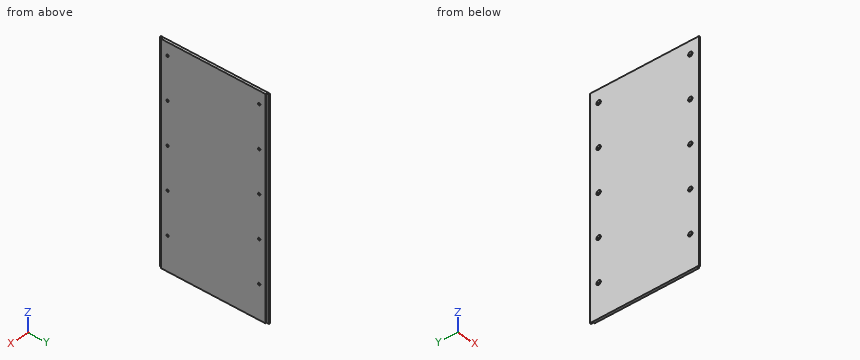
from build123d import *

# Parameters (mm, degrees)
SKETCH1_W                                            = 510
SKETCH1_H                                            = 260
BOSS_EXTRUDE1_DEPTH                                  = 6
SKIZZE2_W                                            = 3
SKIZZE2_H                                            = 6
SCHNITT_LINEAR_AUSTRAGEN1_DEPTH                      = 527.34209408
CSK_FOR_M5_COUNTERSUNK_RAISED_HEAD_SCREW_D           = 5.5
CSK_FOR_M5_COUNTERSUNK_RAISED_HEAD_SCREW_CSINK_D     = 10.4
CSK_FOR_M5_COUNTERSUNK_RAISED_HEAD_SCREW_CSINK_ANGLE = 90
LPATTERN1_COUNT                                      = 5
LPATTERN1_PITCH                                      = 100
MIRROR1_COPY_1_D                                     = 5.5
MIRROR1_COPY_1_CSINK_D                               = 10.4
MIRROR1_COPY_1_CSINK_ANGLE                           = 90
MIRROR1_COPY_2_D                                     = 5.5
MIRROR1_COPY_2_CSINK_D                               = 10.4
MIRROR1_COPY_2_CSINK_ANGLE                           = 90
MIRROR1_COPY_3_D                                     = 5.5
MIRROR1_COPY_3_CSINK_D                               = 10.4
MIRROR1_COPY_3_CSINK_ANGLE                           = 90
MIRROR1_COPY_4_D                                     = 5.5
MIRROR1_COPY_4_CSINK_D                               = 10.4
MIRROR1_COPY_4_CSINK_ANGLE                           = 90


with BuildPart() as part:
    # Sketch1 → Boss-Extrude1 (new body)
    with BuildSketch(Plane(origin=(0, 0, 0), x_dir=(0, 0, -1), z_dir=(1, 0, 0))):
        Rectangle(SKETCH1_W, SKETCH1_H)
    extrude(amount=BOSS_EXTRUDE1_DEPTH)

    # Skizze2 → Schnitt-Linear austragen1 (cut, through all)
    with BuildSketch(Plane.XY.offset(255)):
        with Locations((4.5, 127)):
            Rectangle(SKIZZE2_W, SKIZZE2_H)
        with Locations((4.5, -127)):
            Rectangle(SKIZZE2_W, SKIZZE2_H)
    extrude(amount=-SCHNITT_LINEAR_AUSTRAGEN1_DEPTH, mode=Mode.SUBTRACT)

    # CSK for M5 Countersunk Raised Head Screw1 (through all)
    with Locations(Plane.ZY):
        with Locations((225, -109)):
            csk_for_m5_countersunk_raised_head_screw = CounterSinkHole(CSK_FOR_M5_COUNTERSUNK_RAISED_HEAD_SCREW_D / 2, CSK_FOR_M5_COUNTERSUNK_RAISED_HEAD_SCREW_CSINK_D / 2, counter_sink_angle=CSK_FOR_M5_COUNTERSUNK_RAISED_HEAD_SCREW_CSINK_ANGLE)

    # LPattern1: CSK for M5 Countersunk Raised Head Screw1 ×5
    with Locations(*[(0, 0, -i * LPATTERN1_PITCH) for i in range(1, LPATTERN1_COUNT)]):
        add(csk_for_m5_countersunk_raised_head_screw, mode=Mode.SUBTRACT)

    # Mirror1: CSK for M5 Countersunk Raised Head Screw1 across plane
    add(csk_for_m5_countersunk_raised_head_screw.mirror(Plane.ZX), mode=Mode.SUBTRACT)

    # Mirror1 copy 1 (through all)
    with Locations(Plane(origin=(0, 0, -100), x_dir=(0, 0, 1), z_dir=(-1, 0, 0))):
        with Locations((225, 109)):
            CounterSinkHole(MIRROR1_COPY_1_D / 2, MIRROR1_COPY_1_CSINK_D / 2, counter_sink_angle=MIRROR1_COPY_1_CSINK_ANGLE)

    # Mirror1 copy 2 (through all)
    with Locations(Plane(origin=(0, 0, -200), x_dir=(0, 0, 1), z_dir=(-1, 0, 0))):
        with Locations((225, 109)):
            CounterSinkHole(MIRROR1_COPY_2_D / 2, MIRROR1_COPY_2_CSINK_D / 2, counter_sink_angle=MIRROR1_COPY_2_CSINK_ANGLE)

    # Mirror1 copy 3 (through all)
    with Locations(Plane(origin=(0, 0, -300), x_dir=(0, 0, 1), z_dir=(-1, 0, 0))):
        with Locations((225, 109)):
            CounterSinkHole(MIRROR1_COPY_3_D / 2, MIRROR1_COPY_3_CSINK_D / 2, counter_sink_angle=MIRROR1_COPY_3_CSINK_ANGLE)

    # Mirror1 copy 4 (through all)
    with Locations(Plane(origin=(0, 0, -400), x_dir=(0, 0, 1), z_dir=(-1, 0, 0))):
        with Locations((225, 109)):
            CounterSinkHole(MIRROR1_COPY_4_D / 2, MIRROR1_COPY_4_CSINK_D / 2, counter_sink_angle=MIRROR1_COPY_4_CSINK_ANGLE)


solid = part.part
Input: part model. Units: mm. Frame: model coordinates. Round coordinates to 2 decimals unless told otherwise and drop trailing zeros. Loops run counter-clockwise (first coordinate to the right, second up) from the corner with the lowest first, then second, coordinate; pieces in that order, holes last. Notation, with made-up numbers: M 24,48 L 71,48 A23 ccw 71,56 Z; hole C -18,59.5 d1. An arc over 180 degrees is marked long. Answer as CSV lines item,"result". Start each with the question number.
(1) Line query: line 1 (Y direction, x = 3.75, z = 25); line 2 (Z direction, x = 4.1, y = -109); line 3 (Y direction, x = 4.6, z = -189). Output: solid intervals per line, ascending. Write a range as [from, to].
(2) First-contact query: pin 1 (9 mm diameter, centred on y = 109, z = 25, fed in from -X); pin 2 (6.5 mm diameter, centred on y = 109, z = 125, fed in from -X); pin 3 (3.5 mm diameter, centred on y = -109, z = -175, fed in from +X); pin 4 (1.8 mm diameter, centred on y = 127, z = -104.5, fed in from +X). Flat tips, straight axial feed; report the tip coordinate or a pass-through.
(3) Section A-A, the plane z = 75.5. Output: boundary loops of the cut face in (x, y).
Values found:
1,line 1,"y = [-124, -111.75], [-106.25, 106.25], [111.75, 124]"
1,line 2,"z = [-255, -177.75], [-172.25, -77.75], [-72.25, 22.25], [27.75, 122.25], [127.75, 222.25], [227.75, 255]"
1,line 3,"y = [-124, 124]"
2,pin 1,"stops at x = 0.7"
2,pin 2,"stops at x = 1.95"
2,pin 3,"passes through"
2,pin 4,"stops at x = 3"
3,outline,"M 0,-130 L 3,-130 L 3,-124 L 6,-124 L 6,124 L 3,124 L 3,130 L 0,130 Z"
